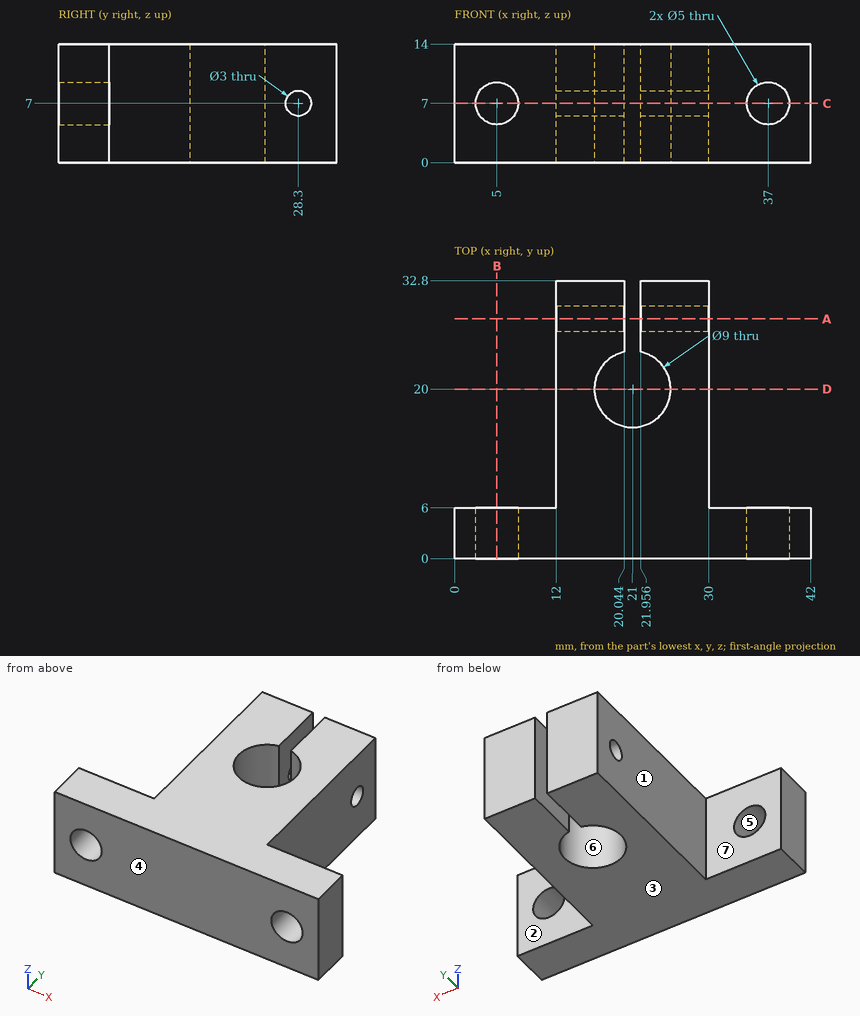
For this review, use the dimensioned drawing (mm, ordinates from the lowest corner) and the shaded views. A direction names the side the tool comes from. Round coordinates to 2 decimals unless told otherwise and drop trailing zeros. Write each loop counter-clockwise with the first axis right and the second up, starting at its lowest first coordinate (ties: lowest second). Pieces come first, ordered by that corner, then holes. Notation, with made-up numbers: M 26.25,-13.5 L 81.25,-13.5 A18 cw 81.25,8.5 Z; hole C 38,27 d5. An arc over 180 degrees is marked long. Write item = value, one per line. Start each with the question number.
(1) We need section B-B (x = 5). Give the boundary of the cut face in (y, z), then the cut area to 3 significant figures.
(2) The part is to be moulded in two halves that separate along Y. For the marked faces 4, 5, 6 and 7, say which applies: +Y half, -Y half, draft (parallel to the pull), parting line (faces both ways), or undercut.
(3) For the marked faces 1, 2 and 3, list the 3-axis set-ups (+Z, -Z, +X, -X, +Y, -Y) from which the entire face can be reached by the end or side of a thin tool; tool diameter is ignored.
(4) For line 1 along X through (y, z) = (4.45, 7); line 2 along X through (y, z) = (31.5, 11); line 3 along X through (y, z) = (20, 7), list the stretches that pass through material, from the lowest coordinate up.
(5) We need section C-C (z = 7). Give the boundary of the cut face in (x, y).
(6) We need section A-A (y = 28.3). Give the boundary of the cut face in (x, z), then the cut area to 3 significant figures.
(7) We need section D-D (y = 20). Give the boundary of the cut face in (x, z).
(8) Clearance check with flat-ended pins moving along their axes: pin 1 Ø2 at (x, z) = (9.5, 8.5) entering from +Y; pin 2 Ø2.5 at (y, z) = (29.5, 8) entering from -X; pin 3 Ø1.5 at (y, z) = (16, 12) entering from +X; pin 4 Ø4.5 at (x, z) = (5, 7) entering from -Y. State where each tip first meets the part, or that it passes through.
Results found:
q1.outline = M 0,0 L 6,0 L 6,4.5 L 0,4.5 Z; M 0,9.5 L 6,9.5 L 6,14 L 0,14 Z
q1.area = 54.0 mm²
q2.face_4 = -Y half
q2.face_5 = draft
q2.face_6 = undercut
q2.face_7 = +Y half
q3.face_1 = +Z, -Z, -X, +Y
q3.face_2 = +Z, -Z, +X, +Y
q3.face_3 = -Z, +X, -X, +Y, -Y
q4.line_1 = 0 to 2.5, 7.5 to 34.5, 39.5 to 42
q4.line_2 = 12 to 20.04, 21.96 to 30
q4.line_3 = 12 to 16.5, 25.5 to 30
q5.outline = M 0,0 L 2.5,0 L 2.5,6 L 0,6 Z; M 7.5,0 L 34.5,0 L 34.5,6 L 30,6 L 30,26.8 L 21.96,26.8 L 21.96,24.4 A4.5 cw long 20.04,24.4 L 20.04,26.8 L 12,26.8 L 12,6 L 7.5,6 Z; M 12,29.8 L 20.04,29.8 L 20.04,32.8 L 12,32.8 Z; M 21.96,29.8 L 30,29.8 L 30,32.8 L 21.96,32.8 Z; M 39.5,0 L 42,0 L 42,6 L 39.5,6 Z
q6.outline = M 12,0 L 20.04,0 L 20.04,5.5 L 12,5.5 Z; M 12,8.5 L 20.04,8.5 L 20.04,14 L 12,14 Z; M 21.96,0 L 30,0 L 30,5.5 L 21.96,5.5 Z; M 21.96,8.5 L 30,8.5 L 30,14 L 21.96,14 Z
q6.area = 177 mm²
q7.outline = M 12,0 L 16.5,0 L 16.5,14 L 12,14 Z; M 25.5,0 L 30,0 L 30,14 L 25.5,14 Z
q8.pin_1 = 6
q8.pin_2 = 12
q8.pin_3 = 30
q8.pin_4 = through
